Here's the drawing with two shaded views (mm, measured from the low corner). I have some questions. A direction names the side the tool comes from. Round coordinates to 2 decimals unless told otherwise and drop trailing zeros. Write each loop counter-clockwise with the first axis right and the second up, starting at its lowest first coordinate (ties: lowest second). Pieces come first, ordered by that corner, then holes. Notation, with made-up numbers: M -27.75,28.5 L -3.75,28.5 A31 ccw -3.75,59.5 Z; hole C 27,25.5 d11. An arc over 180 degrees is marked long. Answer as a JSON object with one key per item and string values. Group by question number.
1) Please list where these lines run through material, in increasing order: L1, parallel to Y at x = 13, z = 1; L2, parallel to Z at x = 34, y = 10. Write a range as [from, to].
2) Suppose I cut it at A-A, the plane y = 18. Write out the boundary of the cut face in (x, z).
3) Suppose I cut it at B-B, the plane z = 28. Write out the boundary of the cut face in (x, y).
4) Suppose I cut it at D-D, the plane x = 26. Write out the boundary of the cut face in (y, z).
5) Suppose I cut it at C-C, the plane x = 33. Write out the boundary of the cut face in (y, z).
6) I'm going to push flat-ended pins straight in: pin 1 Ø4 at (x, y) = (13.5, 15.5) entering from +Z; pin 2 Ø8 at (x, y) = (28, 11.5) entering from +Z; pin 3 Ø12 at (x, z) = (15.5, 18.5) entering from +Y. Where does each tip first touch, or does it pass through?
7) On a 3-axis mill with a long thin cutter (end or side, diameter ignored), from which of +Z, -Z, +X, -X, +Y, -Y can I reach the whole of each face in a straight line? I mean the marked faces 1 and 2. Say none if no direction works.
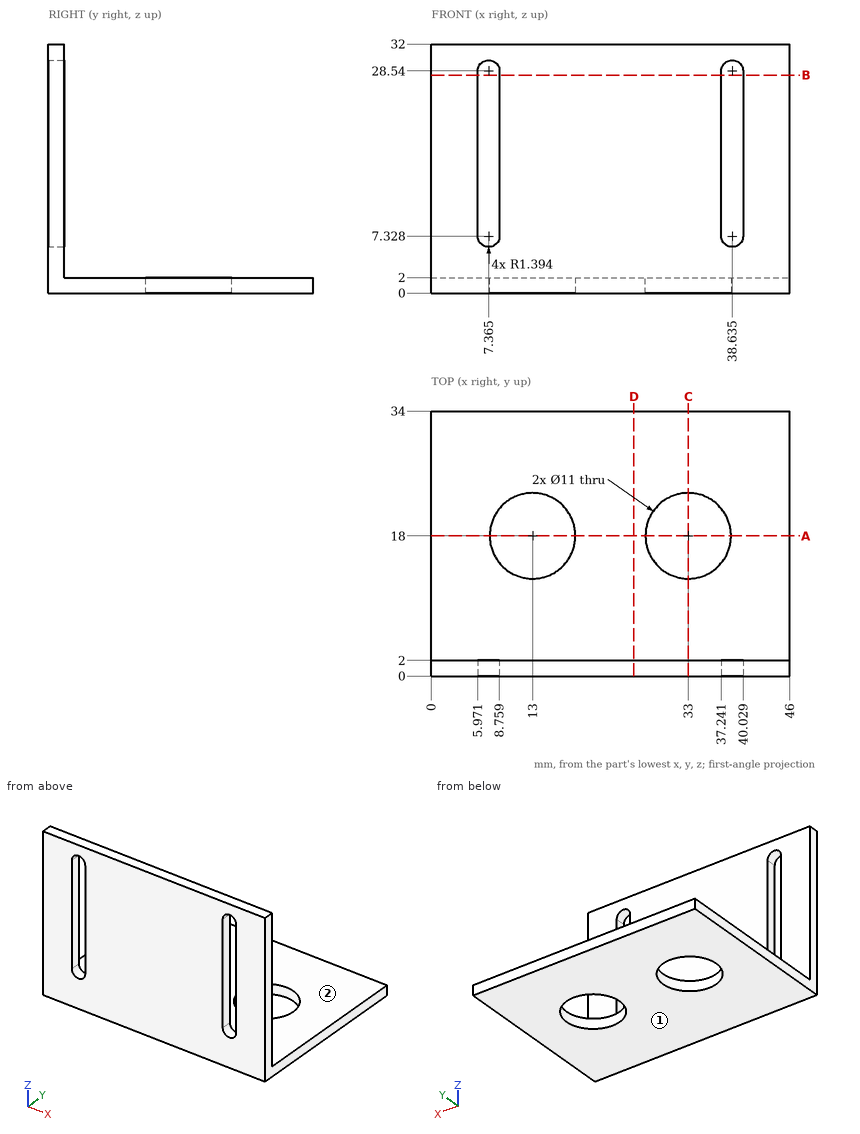
Results:
{
 "1": {"L1": "[0, 12.5], [23.5, 34]", "L2": "[0, 2]"},
 "2": {"outline": "M 0,0 L 7.5,0 L 7.5,2 L 0,2 Z; M 18.5,0 L 27.5,0 L 27.5,2 L 18.5,2 Z; M 38.5,0 L 46,0 L 46,2 L 38.5,2 Z"},
 "3": {"outline": "M 0,0 L 5.97,0 L 5.97,2 L 0,2 Z; M 8.76,0 L 37.24,0 L 37.24,2 L 8.76,2 Z; M 40.03,0 L 46,0 L 46,2 L 40.03,2 Z"},
 "4": {"outline": "M 0,0 L 34,0 L 34,2 L 2,2 L 2,32 L 0,32 Z"},
 "5": {"outline": "M 0,0 L 12.5,0 L 12.5,2 L 2,2 L 2,32 L 0,32 Z; M 23.5,0 L 34,0 L 34,2 L 23.5,2 Z"},
 "6": {"pin 1": "through", "pin 2": "z = 2", "pin 3": "y = 2"},
 "7": {"face 1": "-Z, +X, -X, +Y, -Y", "face 2": "+Z, +X, -X, +Y"}
}
